Read the model definition and answer for the solid it produces. Units are mm, in the model's axes. Give positions to 0.01 mm unless a question says otherwise; leave off trailing zeros. Loops run counter-clockwise (first coordinate to the right, second up) from the corner with the lowest first, then second, coordinate; pieces in that order, holes last. Notation, with made-up numbers: (61, 41) - (86, 41) arc R20 ccw to (86, 63) - close; hole circle Ø9 at (-6.75, -27). An arc over 180 degrees is marked (long way). Put each result on its own line as item: value. Start each with the question number.
1. A cutting plane is placed at A-A, the plane z = 0. Determine the outline of the cut face in (x, y), plus the area to 3 significant figures.
2. Consider L1, parallel to Z at x = 0, y = -6.25; L2, parallel to X at y = -0.75, z = 2.5; L3, parallel to X at y = -4, z = -2.75. Determine where each line is inside the solid, lowest interval first. Write a range as from..to.
3. A cutting plane is placed at C-C, the plane x = -3.25. Determine the outline of the cut face in (y, z), plus the area to 3 significant figures.
4. For a pull along Z with two mould halves and no side action, classify faces 1 (the cylindrical face through (-3, -5, 0)), 2 (the cylindrical face through (-4.197, -5.523, -1.322)), 3 (the flat face through (1, -13.128, 3)) as released by +Z, released by -Z, zero draft, split by the parting line, or undercut.
5. A cutting plane is placed at D-D, the plane y = 1. Determine the outline of the cut face in (x, z).
6. Given pin 1 Ø1 at (x, y) = (2, -1) entering from +Z; pin 2 Ø1.5 at (y, z) = (-8, -2.5) entering from -X; pin 3 Ø2 at (y, z) = (-8, -3.5) entering from +X, each flat-ended and moving along its own axis, determine where each tip first touches the part or whether it passes through.
7. A cutting plane is placed at B-B, the plane x = 0. Determine the outline of the cut face in (y, z), plus the area to 3 significant figures.
```python
from build123d import *

# Parameters (mm, degrees)
SKETCH4_R           = 3
BOSS_EXTRUDE1_DEPTH = 16
SKETCH5_R           = 3
CUT_EXTRUDE1_DEPTH  = 16


with BuildPart() as part:
    # Sketch2 → Revolve3 (revolve)
    with BuildSketch(Plane.XY):
        Polygon((-5, 2.872057786), (0, 2.872057786), (0, -13.127942214), (-4.4, -13.127942214), (-4.4, 1.872057786), (-5, 1.872057786), align=None)
    revolve(axis=Axis((0, 2.872057786, 0), (0, -1, 0)))

    # Sketch4 → Boss-Extrude1 (add)
    with BuildSketch(Plane.XZ.offset(13.127942214)):
        Circle(SKETCH4_R)
    extrude(amount=-BOSS_EXTRUDE1_DEPTH)

    # Sketch5 → Cut-Extrude1 (cut)
    with BuildSketch(Plane.XZ.offset(13.127942214)):
        Circle(SKETCH5_R)
    extrude(amount=-CUT_EXTRUDE1_DEPTH, mode=Mode.SUBTRACT)


solid = part.part
```
Return value:
1. outline: (-5, 1.87) - (-4.4, 1.87) - (-4.4, -13.13) - (-3, -13.13) - (-3, 2.87) - (-5, 2.87) - close; (3, -13.13) - (4.4, -13.13) - (4.4, 1.87) - (5, 1.87) - (5, 2.87) - (3, 2.87) - close
1. area: 46.0 mm2
2. L1: z = -4.4..-3, 3..4.4
2. L2: x = -3.62..-1.66, 1.66..3.62
2. L3: x = -3.43..-1.2, 1.2..3.43
3. outline: (-13.13, -2.97) - (1.87, -2.97) - (1.87, -3.8) - (2.87, -3.8) - (2.87, 3.8) - (1.87, 3.8) - (1.87, 2.97) - (-13.13, 2.97) - close
3. area: 96.6 mm2
4. face 1: undercut
4. face 2: split by the parting line
4. face 3: zero draft
5. outline: circle Ø8.8 at (0, 0); hole circle Ø6 at (0, 0)
6. pin 1: stops at z = 4.14
6. pin 2: stops at x = -4.04
6. pin 3: stops at x = 3.62
7. outline: (-13.13, -4.4) - (1.87, -4.4) - (1.87, -5) - (2.87, -5) - (2.87, -3) - (-13.13, -3) - close; (-13.13, 3) - (2.87, 3) - (2.87, 5) - (1.87, 5) - (1.87, 4.4) - (-13.13, 4.4) - close
7. area: 46.0 mm2
